Can you work these out from the drawing? Everything is in mm from the part's minimum corner. A direction names the side the tool comes from. Coordinates: 2 decimals unless noted, no trailing zeros. Order: outer loops, then holes, each group sorted by start corner. A loop starts at its lowest first (then second) coordinate and runs counter-clockwise, first axis right, second up. Notation, with made-up numbers: (-3, 15) -> (43, 15) arc R18 cw to (43, 37) -> close; hole circle Ø1 at (-32.75, 18). An arc over 180 degrees is marked (long way). Return JSON: item names as keys, results as strings. Group by question number.
1) If we section it at A-A, the plane y = 8: Please give me the cut outline in (x, z), then the cut area to 3 significant figures.
2) If we section it at C-C, the plane x = 7.5: Please give me the cut outline in (y, z).
3) If we section it at B-B, the plane z = 9.75: Please give me the cut outline in (x, y), then the cut area to 3 significant figures.
4) For the marked faces 1 and 2, which set-ups out of +Z, -Z, +X, -X, +Y, -Y let a thin tool reach every point of the face, with its end or its side?
5) For pin 1 (3 mm diameter, centred on y = 20, z = 4.5, fed in from +X); pin 2 (4.5 mm diameter, centred on x = 7, z = 8, fed in from +Y); pin 3 (1 mm diameter, centred on x = 14, z = 10, fed in from +Y), each with a flat end and sliding along its axis, tell me the tip position at first contact or that it passes through.
6) Thinking about a two-plate mould opening in X: for the marked faces 3, 4 and 5, which applies, +X half, -X half, draft (parallel to the pull), parting line (faces both ways), or undercut?
7) If I drill on probe 1 along X at (y, z) = (13, 12); probe 2 along Y at (x, z) = (8.25, 14.25), over which ranges is the centre line in solid material (lowest first)? Write a range as from..to.
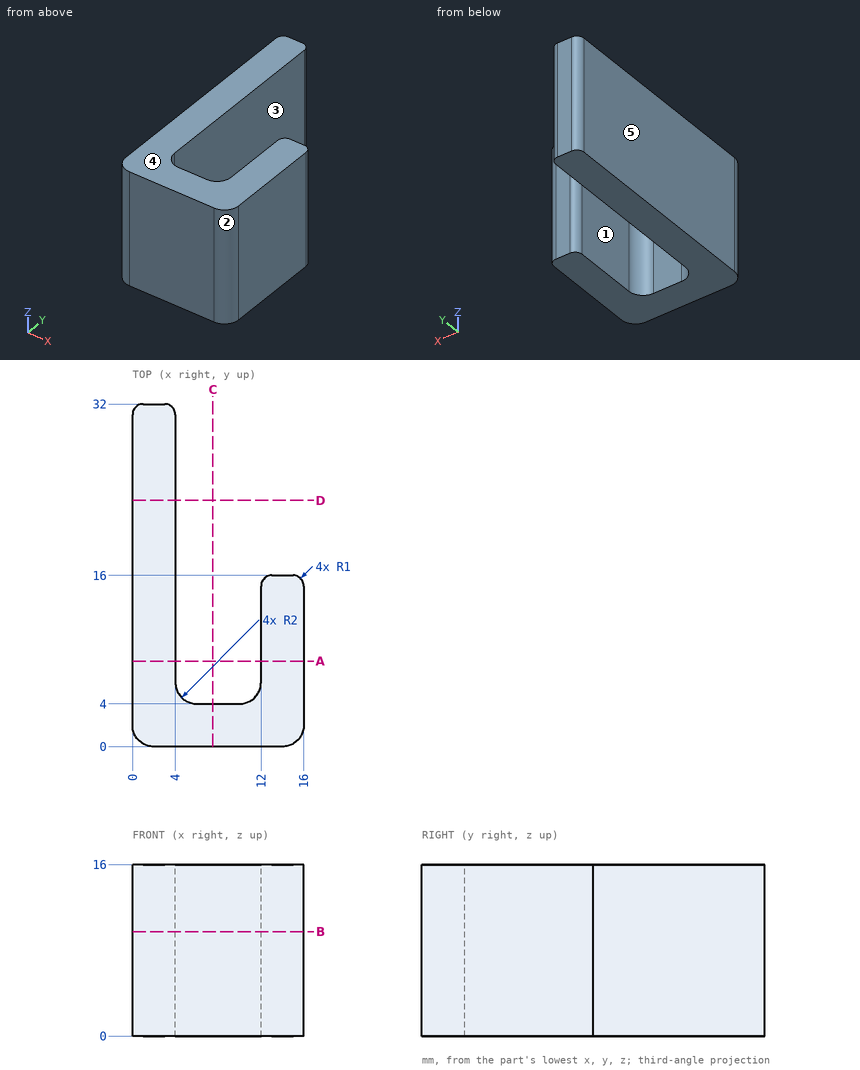
Result sheet:
{
 "1": {"outline": "(0, 0) -> (4, 0) -> (4, 16) -> (0, 16) -> close; (12, 0) -> (16, 0) -> (16, 16) -> (12, 16) -> close", "area": "128 mm2"},
 "2": {"outline": "(0, 0) -> (4, 0) -> (4, 16) -> (0, 16) -> close"},
 "3": {"outline": "(0, 2) arc R2 ccw to (2, 0) -> (14, 0) arc R2 ccw to (16, 2) -> (16, 15) arc R1 ccw to (15, 16) -> (13, 16) arc R1 ccw to (12, 15) -> (12, 6) arc R2 cw to (10, 4) -> (6, 4) arc R2 cw to (4, 6) -> (4, 31) arc R1 ccw to (3, 32) -> (1, 32) arc R1 ccw to (0, 31) -> close", "area": "223 mm2"},
 "4": {"face 1": "+Z, -Z, +Y", "face 2": "+Z, -Z, +X, -Y"},
 "5": {"pin 1": "stops at x = 4", "pin 2": "stops at y = 4.44", "pin 3": "stops at y = 16"},
 "6": {"face 3": "undercut", "face 4": "draft", "face 5": "-X half"},
 "7": {"probe 1": "x = 0..4, 12..16", "probe 2": "y = 0..4"}
}
